Part model, mm, in its own coordinate system. A direction names the side the tool comes from. Give positions to 0.01 mm unless a question says otherwise; leave off trailing zeros. Order: outer loops, then holes, each group sorted by start corner. A loop starts at its lowest first (then second) coordinate and runs counter-clockwise, first axis right, second up. Notation, with made-up numbers: M -15,85 L 38,85 A32 cw 38,112 Z; hole C -3.5,17 d7. An arc over 180 degrees is marked long. Answer as a JSON object with one key per item and string values.
from build123d import *

# Parameters (mm, degrees)
SKETCH3_R           = 9.525
BOSS_EXTRUDE1_DEPTH = 25.4
SKETCH5_R           = 3.556
CUT_EXTRUDE1_DEPTH  = 43.121134838
SKETCH6_R           = 6.35
CUT_EXTRUDE2_DEPTH  = 5.08
CUT_EXTRUDE2_DRAFT  = -31
SKETCH7_R           = 1.397
CUT_EXTRUDE3_DEPTH  = 39.1


with BuildPart() as part:
    # Sketch2 → Revolve2 (revolve)
    with BuildSketch(Plane.XY):
        with BuildLine():
            Line((12.7, 0), (0, 0))
            Line((0, 0), (0, 12.7))
            ThreePointArc((0, 12.7), (8.980256121, 8.980256121), (12.7, 0))
        make_face()
    revolve(axis=Axis((0, 67.537553081, 0), (0, -1, 0)))

    # Sketch3 → Boss-Extrude1 (add)
    with BuildSketch(Plane.XZ):
        with Locations(Location((0, 0, 0), (0, 0, 90))):
            Circle(SKETCH3_R)
    extrude(amount=BOSS_EXTRUDE1_DEPTH)

    # Sketch5 → Cut-Extrude1 (cut, through all)
    with BuildSketch(Plane.XZ.offset(25.4)):
        with Locations(Location((0, 0, 0), (0, 0, 270))):
            Circle(SKETCH5_R)
    extrude(amount=-CUT_EXTRUDE1_DEPTH, mode=Mode.SUBTRACT)


with BuildPart() as cut_extrude2_tool:
    # Sketch6 → Cut-Extrude2 (with draft: the straight prism first)
    with BuildSketch(Plane(origin=(0, 12.7, 0), x_dir=(1, 0, 0), z_dir=(0, 1, 0))):
        Circle(SKETCH6_R)
    extrude(amount=-CUT_EXTRUDE2_DEPTH)
    # Cut-Extrude2: the draft: its side faces are tilted about the plane it starts from
    cut_extrude2_sides = [cut_extrude2_tool.faces().sort_by_distance(p)[0] for p in [
        (-6.35, 10.16, 0),
    ]]
    draft(cut_extrude2_sides, Plane(origin=(0, 12.7, 0), x_dir=(1, 0, 0), z_dir=(0, 1, 0)), CUT_EXTRUDE2_DRAFT)


with BuildPart() as part_1:
    add(part.part)

    # Cut-Extrude2: cut by cut_extrude2_tool
    add(cut_extrude2_tool.part, mode=Mode.SUBTRACT)

    # Sketch7 → Cut-Extrude3 (cut, through all)
    with BuildSketch(Plane.XY.offset(12.7)):
        with Locations((0, -19.05)):
            Circle(SKETCH7_R)
    extrude(amount=-CUT_EXTRUDE3_DEPTH, mode=Mode.SUBTRACT)


solid = part_1.part
1. Cut at C-C on y = -19.05. Give the cut face in (x, z) (3 decimals), plus the area to 3 significant figures.
Worked answers:
{"outline": "M -1.397,-9.422 L -1.397,-3.27 A3.556 cw -1.397,3.27 L -1.397,9.422 A9.525 ccw Z; M 1.397,-9.422 A9.525 ccw 1.397,9.422 L 1.397,3.27 A3.556 cw 1.397,-3.27 Z", "area": "212 mm^2"}
2. Cut at B-B on x = 0. Give the cut face in (y, z) (3 decimals).
Worked answers:
{"outline": "M -25.4,-9.525 L -20.447,-9.525 L -20.447,-3.556 L -25.4,-3.556 Z; M -25.4,3.556 L -20.447,3.556 L -20.447,9.525 L -25.4,9.525 Z; M -17.653,-9.525 L 0,-9.525 L 0,-12.7 A12.7 ccw 11.411,-5.575 L 8.05,-3.556 L -17.653,-3.556 Z; M -17.653,3.556 L 8.05,3.556 L 11.411,5.575 A12.7 ccw 0,12.7 L 0,9.525 L -17.653,9.525 Z"}
3. Cut at A-A on z = 0. Give the cut face in (x, y) (3 decimals).
Worked answers:
{"outline": "M -12.7,0 L -9.525,0 L -9.525,-25.4 L -3.556,-25.4 L -3.556,8.05 L -5.575,11.411 A12.7 ccw Z; M 3.556,-25.4 L 9.525,-25.4 L 9.525,0 L 12.7,0 A12.7 ccw 5.575,11.411 L 3.556,8.05 Z"}
4. Two-plate mould, pull along Y, no slides. Class faces 3 (the conical face through (-0.798, 8.26, 3.595)), 4 (the cylindrical face through (-1.362, -8.909, -3.285)), 5 (the cylindrical face through (-0.182, -17.665, -6.355)): +Y half, -Y half, draft (parallel to the pull), parting line (faces both ways), or undercut.
Worked answers:
{"face 3": "+Y half", "face 4": "draft", "face 5": "undercut"}
5. Probe line 1 along X through (y, z) = (-15, 0) (3 decimals); line 2 along Z through (x, y) = (-1.5, 3); line 3 along Z through (x, y) = (2.25, -8). List the from-to ranges inside material, lowest first.
Worked answers:
{"line 1": "x = -9.525 to -3.556, 3.556 to 9.525", "line 2": "z = -12.25 to -3.22, 3.22 to 12.25", "line 3": "z = -9.26 to -2.75, 2.75 to 9.26"}
6. Which spindle directions (+Z, -Z, +X, -X, +Y, -Y) get a long thin tool onto all of the face, cutting with end or side? Do faces 1 (the flat face through (5, 0, 9)), 2 (the cylindrical face through (-0.182, -17.665, 6.441)). Say none if no direction does.
Worked answers:
{"face 1": "-Y", "face 2": "+Z, -Z"}
7. Pin check, flat tips, straight feed: P1, Ø4, axis at y = -19.5, z = -5.5, coming from the +X side; P2, Ø2, axis at x = 5, z = -8.5, coming from the -Y side; P3, Ø1, axis at y = -15, z = -3.5, coming from the +X side; P4, Ø3.5, axis at x = 0, y = -19.05, coming from the -Z side (3 decimals). Stop position of each tip, or through.
Worked answers:
{"P1": "stops at x = 8.86", "P2": "stops at y = -25.4", "P3": "stops at x = 9.04", "P4": "stops at z = -9.525"}
8. Cut at D-D on y = -15. Give the cut face in (x, z) (3 decimals).
Worked answers:
{"outline": "C 0,0 d19.05; hole C 0,0 d7.112"}
